Work out the finished part from the listing and answer in its coordinate system (mm). Face numbers are marked on the shaded views. Coordinates: 2 decimals unless noted, no trailing zeros. Order: outer loops, then holes, each group sorted by start corner. A loop starts at its lowest first (then second) coordinate and runs counter-clockwise, first axis right, second up. Notation, with made-up numbers: M 5.25,29.25 L 33.25,29.25 A10 cw 33.25,44.25 Z; hole C 63,2.5 d10. An arc over 180 degrees is marked long. Use a Markdown table: item, result.
from build123d import *

# Parameters (mm, degrees)
F1_DEPTH = 60


with BuildPart() as f1:
    # F0 (on Right) → F1 (new body, symmetric)
    with BuildSketch(Plane.YZ):
        with BuildLine():
            ThreePointArc((-3.824065, -4.623475), (-2.554957, 5.42883), (6, 0))
            ThreePointArc((6, 0), (5.42883, -2.554957), (3.824065, -4.623475))
            Line((3.824065, -4.623475), (6.928203, -10))
            Line((6.928203, -10), (15, -10))
            Line((15, -10), (15, 10))
            Line((15, 10), (-15, 10))
            Line((-15, 10), (-15, -10))
            Line((-15, -10), (-6.928203, -10))
            Line((-6.928203, -10), (-3.824065, -4.623475))
        make_face()
    extrude(amount=F1_DEPTH, both=True)


solid = f1.part
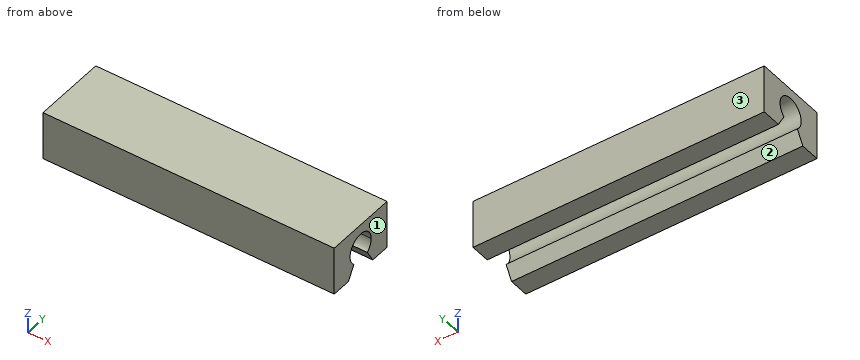
1. Section A-A on x = 52 is taken. Determine the outline of the cut face in (y, z), then the cut area to 3 significant figures.
Answers below:
| item | result |
|---|---|
| outline | M -15,-10 L -6.93,-10 L -3.82,-4.62 A6 cw long 6,0 A6 cw 3.82,-4.62 L 6.93,-10 L 15,-10 L 15,10 L -15,10 Z |
| area | 436 mm² |
2. Section B-B on y = 0 is taken. Determine the outline of the cut face in (x, z), then the cut area to 3 significant figures.
Answers below:
| item | result |
|---|---|
| outline | M -60,6 L 60,6 L 60,10 L -60,10 Z |
| area | 480 mm² |
3. Find the intervals of material crossed by probe 1 along Z at (x, y) = (27, 0); probe 2 along Y at (x, z) = (10.5, 2); probe 3 along Y at (x, z) = (-7, -3.5), in increasing order.
Answers below:
| item | result |
|---|---|
| probe 1 | 6 to 10 |
| probe 2 | -15 to -5.66, 5.66 to 15 |
| probe 3 | -15 to -4.87, 4.87 to 15 |
4. A flat-ended cylindrical pin translates along its axis: P1, Ø5, axis at x = 27, y = 0, coming from the -Z side. Find the tip coordinate at first contact, or state that the pin passes through.
Answers below:
| item | result |
|---|---|
| P1 | z = 5.45 |
5. For a pull along Y with two mould halves and no side action, classify the marked faces 1, 2 and 3 as +Y half, -Y half, draft (parallel to the pull), parting line (faces both ways), or undercut.
Answers below:
| item | result |
|---|---|
| face 1 | draft |
| face 2 | undercut |
| face 3 | +Y half |
